Can you work these out from the model? Positions are in its coordinate system, mm. A direction names the side the tool comes from. Give positions to 0.01 mm unless a question says otherwise; leave off trailing zeros. Order: outer loops, then holes, each group sorted by start corner. A loop starts at its lowest first (then second) coordinate and runs counter-clockwise, first axis right, second up. Notation, with made-up numbers: M 64,-37.5 L 105,-37.5 A20 ccw 105,-15.5 Z; hole C -17.75,30 d8. An arc over 180 degrees is marked long. Use one line per item in the form item = value. Start each with the question number.
1. We'd pull the mould along X, two halves only. Please class faces 4 (the face through (42, 12, 6)), 5 (the face through (42.28, 26.694, 10.493)), 6 (the face through (33, 35, 5)): +X half, -X half, draft (parallel to the pull), parting line (faces both ways), or undercut.
2. I want a section at B-B, the plane x = 9.5. List the corners of the cut face in (y, z) for me, and give its area (3 significant figures).
3. For faces 1 (the face through (35.005, 17.5, 10.5)), 2 (the face through (42, 8.3, 10.5)), 3 (the face through (45, 15.75, 6)), which set-ups out of +Z, -Z, +X, -X, +Y, -Y let a thin tool reach every point of the face, with its end or its side?
4. I want a section at D-D, the plane x = 42. List the corners of the cut face in (y, z) for me.
5. I need wall thicknesses on L1, parallel to X at y = 17, z = 2.25; L2, parallel to Y at x = 17.5, z = 6; L3, parallel to Y at x = 45.5, z = 8.5. Which ranges of each line are inside material? Lowest first, please.
6. Will these pins go through, and if not, where does the flat tip stop? P1, Ø1.5, axis at y = 26.5, z = 8, coming from the -X side; P2, Ø6, axis at x = 9.5, y = 11, coming from the +Z side; P3, Ø4, axis at y = 20.5, z = 8, coming from the -X side.
7. I want a section at C-C, the plane y = 9.5. List the corners of the cut face in (x, z) for me.
8. I want a section at A-A, the plane z = 8.25. List the corners of the cut face in (x, y) for me, and give its area (3 significant figures).
```python
from build123d import *

# Parameters (mm, degrees)
F0_R     = 12.5
F1_DEPTH = 10
F3_DEPTH = 1
F4_DEPTH = 9


with BuildPart() as f1:
    # F0 (on Top) → F1 (new body)
    with BuildSketch(Plane.XY):
        with BuildLine():
            ThreePointArc((0, 17.5), (5.1256313292, 5.1256313292), (17.5, 0))
            Line((17.5, 0), (49, 0))
            ThreePointArc((49, 0), (52.5355339059, 1.4644660941), (54, 5))
            Line((54, 5), (54, 30))
            ThreePointArc((54, 30), (52.5355339059, 33.5355339059), (49, 35))
            Line((49, 35), (17.5, 35))
            ThreePointArc((17.5, 35), (5.1256313292, 29.8743686708), (0, 17.5))
        make_face()
        with Locations((17.5, 17.5)):
            Circle(F0_R, mode=Mode.SUBTRACT)
    extrude(amount=F1_DEPTH)

    # F2 (on face) → F3 (join)
    with BuildSketch(Plane.XY.offset(10)):
        with BuildLine():
            ThreePointArc((49, 19.7), (42.1277095354, 26.6988349227), (35.0046599215, 19.9553765589))
            Line((35.0046599215, 19.9553765589), (35.0046599215, 19.4446234411))
            Line((35.0046599215, 19.4446234411), (35.0046599215, 17.5))
            Line((35.0046599215, 17.5), (35.0046599215, 15.5553765589))
            Line((35.0046599215, 15.5553765589), (35.0046599215, 15.0446234411))
            ThreePointArc((35.0046599215, 15.0446234411), (42.1277095354, 8.3011650773), (49, 15.3))
            Line((49, 15.3), (49, 17.5))
            Line((49, 17.5), (49, 19.7))
        make_face()
        Polygon((41, 23), (43, 23), (43, 19.25), (47.25, 19.25), (47.25, 15.75), (43, 15.75), (43, 12), (41, 12), (41, 15.75), (36.75, 15.75), (36.75, 19.25), (41, 19.25), align=None, mode=Mode.SUBTRACT)
    extrude(amount=F3_DEPTH)

    # F4 (cut): a face of the model
    f4_faces = [f1.faces().sort_by_distance(p)[0] for p in [
        (42, 17.5, 10),
    ]]
    extrude(f4_faces, amount=-F4_DEPTH, mode=Mode.SUBTRACT)


solid = f1.part
```
Check result:
q1.face_4 = undercut
q1.face_5 = parting line
q1.face_6 = draft
q2.outline = M 1.94,0 L 7.9,0 L 7.9,10 L 1.94,10 Z; M 27.1,0 L 33.06,0 L 33.06,10 L 27.1,10 Z
q2.area = 119 mm2
q3.face_1 = +Z, -X, +Y, -Y
q3.face_2 = +Z, -Y
q3.face_3 = +Z
q4.outline = M 0,0 L 35,0 L 35,10 L 26.7,10 L 26.7,11 L 23,11 L 23,1 L 12,1 L 12,11 L 8.3,11 L 8.3,10 L 0,10 Z
q5.L1 = 0.01 to 5.01, 29.99 to 36.75, 47.25 to 54
q5.L2 = 0 to 5, 30 to 35
q5.L3 = 0 to 15.75, 19.25 to 35
q6.P1 = 2.07
q6.P2 = 10
q6.P3 = 0.03
q7.outline = M 1.94,0 L 7.9,0 L 7.9,10 L 1.94,10 Z; M 27.1,0 L 54,0 L 54,10 L 45.92,10 L 45.92,11 L 38.08,11 L 38.08,10 L 27.1,10 Z
q8.outline = M 17.5,0 L 49,0 A5 ccw 54,5 L 54,30 A5 ccw 49,35 L 17.5,35 A17.5 ccw Z; hole C 17.5,17.5 d25; hole M 36.75,15.75 L 41,15.75 L 41,12 L 43,12 L 43,15.75 L 47.25,15.75 L 47.25,19.25 L 43,19.25 L 43,23 L 41,23 L 41,19.25 L 36.75,19.25 Z
q8.area = 1,210 mm2
